from build123d import *

# Parameters (mm, degrees)
SKETCH1_R                      = 2
SKETCH1_R_2                    = 1
BASE_FLANGE1_DEPTH             = 2
EDGE_FLANGE1_STRIP_W           = 9.9304
EDGE_FLANGE1_STRIP_H           = 2
EDGE_FLANGE1_STRIP_CUT_DEPTH   = 312
EDGE_FLANGE1_STRIP_2_W         = 9.9304
EDGE_FLANGE1_STRIP_2_H         = 2
EDGE_FLANGE1_STRIP_CUT_2_DEPTH = 312
EDGE_FLANGE1_DEPTH             = 312
EDGE_FLANGE1_BEND_DEPTH        = 312
SKETCH13_R                     = 1
CUT_EXTRUDE1_DEPTH             = 224.494966386


# Sheet-metal steps are written as plain solids
with BuildPart() as part:
    # Sketch1 → Base-Flange1 (new body)
    with BuildSketch(Plane(origin=(0, 0, 0), x_dir=(0, 1, 0), z_dir=(0, 0, 1))):
        Polygon((185, 62.5), (160, 62.5), (160, 58.5), (156, 58.5), (156, 62.5), (-156, 62.5), (-156, 58.5), (-160, 58.5), (-160, 62.5), (-185, 62.5), (-185, -62.5), (-160, -62.5), (-160, -58.5), (-156, -58.5), (-156, -62.5), (156, -62.5), (156, -58.5), (160, -58.5), (160, -62.5), (185, -62.5), align=None)
        with Locations(Location((-152.48, 47.625, 0), (0, 0, 270))):
            Circle(SKETCH1_R, mode=Mode.SUBTRACT)
        with Locations(Location((-120.73, 47.625, 0), (0, 0, 270))):
            Circle(SKETCH1_R, mode=Mode.SUBTRACT)
        with Locations(Location((-76.28, 47.625, 0), (0, 0, 270))):
            Circle(SKETCH1_R, mode=Mode.SUBTRACT)
        with Locations(Location((-152.48, -47.625, 0), (0, 0, 270))):
            Circle(SKETCH1_R, mode=Mode.SUBTRACT)
        with Locations(Location((-120.73, -47.625, 0), (0, 0, 270))):
            Circle(SKETCH1_R, mode=Mode.SUBTRACT)
        with Locations(Location((-76.28, -47.625, 0), (0, 0, 270))):
            Circle(SKETCH1_R, mode=Mode.SUBTRACT)
        with Locations(Location((54.28, 47.625, 0), (0, 0, 90))):
            Circle(SKETCH1_R, mode=Mode.SUBTRACT)
        with Locations(Location((98.73, 47.625, 0), (0, 0, 90))):
            Circle(SKETCH1_R, mode=Mode.SUBTRACT)
        with Locations(Location((130.48, 47.625, 0), (0, 0, 90))):
            Circle(SKETCH1_R, mode=Mode.SUBTRACT)
        with Locations(Location((130.48, -47.625, 0), (0, 0, 90))):
            Circle(SKETCH1_R, mode=Mode.SUBTRACT)
        with Locations(Location((98.73, -47.625, 0), (0, 0, 90))):
            Circle(SKETCH1_R, mode=Mode.SUBTRACT)
        with Locations(Location((54.28, -47.625, 0), (0, 0, 90))):
            Circle(SKETCH1_R, mode=Mode.SUBTRACT)
        with Locations(Location((-179, 56.5, 0), (0, 0, 270))):
            Circle(SKETCH1_R_2, mode=Mode.SUBTRACT)
        with Locations(Location((-179, -56.5, 0), (0, 0, 270))):
            Circle(SKETCH1_R_2, mode=Mode.SUBTRACT)
        with Locations(Location((179, -56.5, 0), (0, 0, 270))):
            Circle(SKETCH1_R_2, mode=Mode.SUBTRACT)
        with Locations(Location((179, 56.5, 0), (0, 0, 270))):
            Circle(SKETCH1_R_2, mode=Mode.SUBTRACT)
        with Locations(Location((0, 56.5, 0), (0, 0, 270))):
            Circle(SKETCH1_R_2, mode=Mode.SUBTRACT)
        with Locations(Location((0, -56.5, 0), (0, 0, 270))):
            Circle(SKETCH1_R_2, mode=Mode.SUBTRACT)
        with Locations(Location((-167, 56, 0), (0, 0, 270))):
            Circle(SKETCH1_R_2, mode=Mode.SUBTRACT)
        with Locations(Location((-77, 56, 0), (0, 0, 270))):
            Circle(SKETCH1_R_2, mode=Mode.SUBTRACT)
        with Locations(Location((-167, -56, 0), (0, 0, 270))):
            Circle(SKETCH1_R_2, mode=Mode.SUBTRACT)
        with Locations(Location((-77, -56, 0), (0, 0, 270))):
            Circle(SKETCH1_R_2, mode=Mode.SUBTRACT)
        with Locations(Location((55, -56, 0), (0, 0, 90))):
            Circle(SKETCH1_R_2, mode=Mode.SUBTRACT)
        with Locations(Location((145, -56, 0), (0, 0, 90))):
            Circle(SKETCH1_R_2, mode=Mode.SUBTRACT)
        with Locations(Location((55, 56, 0), (0, 0, 90))):
            Circle(SKETCH1_R_2, mode=Mode.SUBTRACT)
        with Locations(Location((145, 56, 0), (0, 0, 90))):
            Circle(SKETCH1_R_2, mode=Mode.SUBTRACT)
    extrude(amount=-BASE_FLANGE1_DEPTH)

    # Edge-Flange1 strip (across the edge) → Edge-Flange1 strip cut (cut)
    with BuildSketch(Plane(origin=(-62.5, 156, 0), x_dir=(1, 0, 0), z_dir=(0, -1, 0))):
        with Locations((-2, -1)):
            Rectangle(EDGE_FLANGE1_STRIP_W, EDGE_FLANGE1_STRIP_H)
    extrude(amount=EDGE_FLANGE1_STRIP_CUT_DEPTH, mode=Mode.SUBTRACT)

    # Edge-Flange1 strip 2 (across the edge) → Edge-Flange1 strip cut 2 (cut)
    with BuildSketch(Plane(origin=(62.5, -156, 0), x_dir=(-1, 0, 0), z_dir=(0, 1, 0))):
        with Locations((-2, -1)):
            Rectangle(EDGE_FLANGE1_STRIP_2_W, EDGE_FLANGE1_STRIP_2_H)
    extrude(amount=EDGE_FLANGE1_STRIP_CUT_2_DEPTH, mode=Mode.SUBTRACT)

    # Edge-Flange1 section (across the edge) → Edge-Flange1 (add)
    with BuildSketch(Plane(origin=(-62.5, 156, 0), x_dir=(1, 0, 0), z_dir=(0, -1, 0))):
        with BuildLine():
            Line((0, 0.9652), (0, 10))
            Line((0, 10), (2, 10))
            Line((2, 10), (2, 0.9652))
            ThreePointArc((2, 0.9652), (2.282700535, 0.282700535), (2.9652, 0))
            Line((2.9652, 0), (2.9652, -2))
            ThreePointArc((2.9652, -2), (0.868486972, -1.131513028), (0, 0.9652))
        make_face()
    extrude(amount=EDGE_FLANGE1_DEPTH)

    # Edge-Flange1 section 2 (across the edge) → Edge-Flange1 bend (add)
    with BuildSketch(Plane(origin=(62.5, -156, 0), x_dir=(-1, 0, 0), z_dir=(0, 1, 0))):
        with BuildLine():
            Line((0, 0.9652), (0, 10))
            Line((0, 10), (2, 10))
            Line((2, 10), (2, 0.9652))
            ThreePointArc((2, 0.9652), (2.282700535, 0.282700535), (2.9652, 0))
            Line((2.9652, 0), (2.9652, -2))
            ThreePointArc((2.9652, -2), (0.868486972, -1.131513028), (0, 0.9652))
        make_face()
    extrude(amount=EDGE_FLANGE1_BEND_DEPTH)

    # Sketch13 → Cut-Extrude1 (cut, through all)
    with BuildSketch(Plane.YZ.offset(62.5)):
        with Locations(Location((0, 5, 0), (0, 0, 270))):
            Circle(SKETCH13_R)
        with Locations(Location((150, 5, 0), (0, 0, 270))):
            Circle(SKETCH13_R)
        with Locations(Location((-150, 5, 0), (0, 0, 270))):
            Circle(SKETCH13_R)
    extrude(amount=-CUT_EXTRUDE1_DEPTH, mode=Mode.SUBTRACT)


solid = part.part
Here's how the part is built. I have some questions about the finished solid (model axes, mm). A direction names the side the tool comes from. Give positions to 0.01 mm unless a question says otherwise; leave off trailing zeros. Order: outer loops, then holes, each group sorted by start corner. A loop starts at its lowest first (then second) coordinate and runs counter-clockwise, first axis right, second up. Notation, with made-up numbers: M 66,23 L 101,23 A23 ccw 101,42 Z; hole C -34,88 d6. An arc over 180 degrees is marked long. Answer as a JSON object with one key per item and string values. Group by question number.
1) On a 3-axis mill with a long thin cutter (end or side, diameter ignored), from which of +Z, -Z, +X, -X, +Y, -Y can I reach the whole of each face in a straight line? I mean faces 1 (the flat face through (-62.5, 2, 5)), 2 (the flat face through (60.5, -2, 6)). Say none if no direction works.
2) Suppose I cut it at B-B, the plane x = -1. Write out the boundary of the cut face in (y, z).
3) Please list where these lines run through material, in increasing order: L1, parallel to X at y = 179, z = -0.45; L2, parallel to X at y = -167, z = -1.3; L3, parallel to X at y = 39, z = 4.5. Write a range as [from, to].
4) We'd pull the mould along X, two halves only. Please class faces 3 (the flat face through (62.5, -2, 5)), 4 (the flat face through (-1, -3, -2)), 5 (the flat face through (-60.5, 2, 6)): pulls with the +X half, pulls with the -X half, needs draft (parallel to the pull), parting line crosses it, or undercut.
5) Suppose I cut it at A-A, the plane y = -47. Write out the boundary of the cut face in (x, z).
6) I'm going to push a flat-ended pin straight in: pin 1 Ø5 at (x, y) = (-47.625, -120.73) entering from +Z. Where does the tip first touch, or does it pass through?
Results found:
{
 "1": {"face 1": "+Z, -Z, -X, +Y, -Y", "face 2": "+Z, +Y, -Y"},
 "2": {"outline": "M -185,-2 L 185,-2 L 185,0 L -185,0 Z"},
 "3": {"L1": "[-62.5, -57.5], [-55.5, 55.5], [57.5, 62.5]", "L2": "[-62.5, -57], [-55, 55], [57, 62.5]", "L3": "[-62.5, -60.5], [60.5, 62.5]"},
 "4": {"face 3": "pulls with the +X half", "face 4": "needs draft", "face 5": "undercut"},
 "5": {"outline": "M -62.5,0.97 A2.97 ccw -59.53,-2 L 59.53,-2 A2.97 ccw 62.5,0.97 L 62.5,10 L 60.5,10 L 60.5,0.97 A0.97 cw 59.53,0 L -59.53,0 A0.97 cw -60.5,0.97 L -60.5,10 L -62.5,10 Z"},
 "6": {"pin 1": "z = 0"}
}
